Design review of the part built by this model. Coordinates are the model's own, in mm. Face numbers are marked on the shaded views. A direction names the side the tool comes from. Coordinates: 2 decimals unless noted, no trailing zeros. Write each loop counter-clockwise with the first axis right and the second up, starting at its lowest first coordinate (ties: lowest second). Pieces come first, ordered by that corner, then holes. Notation, with made-up numbers: (85.25, 22.5) - (96.25, 22.5) arc R18 cw to (96.25, 39.5) - close; hole circle Ø8 at (-30.75, -12). An arc over 180 degrees is marked (long way). One line per item, written item: value.
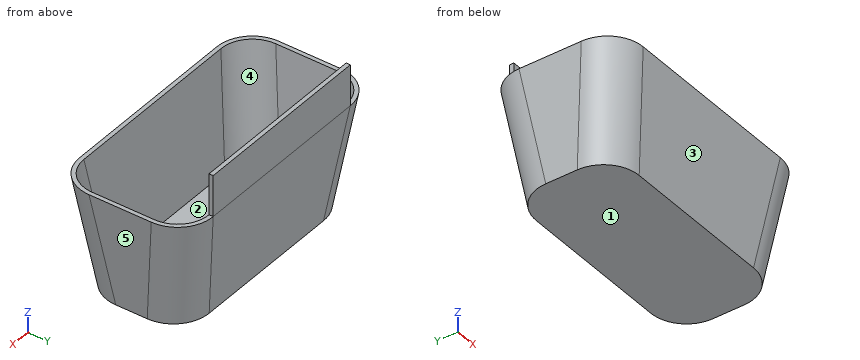
from build123d import *

# Parameters (mm, degrees)
F0_W      = 125
F0_H      = 110
F1_DEPTH  = 65
F3_DEPTH  = 65.001
F5_DEPTH  = 125.001
F8_R      = 35
F9_T      = -4
F10_W     = 180.6418882369
F10_H     = 4.0370187838
F11_DEPTH = 40


with BuildPart() as f1:
    # F0 (on Front) → F1 (new body)
    with BuildSketch(Plane.XZ):
        with Locations((-62.5, 0)):
            Rectangle(F0_W, F0_H)
    extrude(amount=F1_DEPTH)

    # F2 (on face) → F3 (cut, through all)
    with BuildSketch(Plane.XZ.offset(65)):
        Polygon((-110, -55), (-125, 55), (-154.2346477509, 55), (-148.0445983784, -67.179696599), (-108.0001720049, -65.150906356), align=None)
    extrude(amount=-F3_DEPTH, mode=Mode.SUBTRACT)

    # F4 (on face) → F5 (cut, through all)
    with BuildSketch(Plane.YZ):
        Polygon((-50, -55), (-65, 55), (-101.2629643083, 55), (-94.3923816085, -57.4389097095), (-50, -57.4389097095), align=None)
    extrude(amount=-F5_DEPTH, mode=Mode.SUBTRACT)

    # F6: F1 across face


with BuildPart() as f1_1:
    add(f1.part)
    add(f1.part.mirror(Plane(origin=(0, -28.9130434783, 2.3913043478), x_dir=(0, 1, 0), z_dir=(1, 0, 0))))

    # F7: F1 across face


with BuildPart() as f1_2:
    add(f1_1.part)
    add(f1_1.part.mirror(Plane(origin=(0, 0, 1.170212766), x_dir=(-1, 0, 0), z_dir=(0, 1, 0))))

    # F8
    f8_edges = [f1_2.edges().sort_by_distance(p)[0] for p in [
        (-117.5, -57.5, 0),
        (-117.5, 57.5, 0),
        (117.5, -57.5, 0),
        (117.5, 57.5, 0),
    ]]
    fillet(f8_edges, radius=F8_R)

    # F9
    f9_openings = [f1_2.faces().sort_by_distance(p)[0] for p in [
        (0, 0, 55),
    ]]
    offset(amount=F9_T, openings=f9_openings)

    # F10 (on face) → F11 (join)
    with BuildSketch(Plane.XY.offset(55)):
        with Locations((0, 62.9814906081)):
            Rectangle(F10_W, F10_H)
    extrude(amount=F11_DEPTH)


solid = f1_2.part
1. Mouldability with a two-part tool opening along Y and no side actions: class the marked faces 3, 4 and 5 as released by +Y, released by -Y, zero draft, split by the parting line, or undercut.
Answer block:
face 3: released by -Y
face 4: undercut
face 5: zero draft
2. Consider section B-B, the plane z = 61. Write out the cut boundary in (x, y), then the cut area to 3 significant figures.
Answer block:
outline: (-90.32, 60.96) - (90.32, 60.96) - (90.32, 65) - (-90.32, 65) - close
area: 729 mm^2
3. Insertion check: pin 1 Ø2 at (y, z) = (-6, 42) entering from +X; pin 2 Ø3 at (y, z) = (63, 72.5) entering from -X; pin 3 Ø4.5 at (y, z) = (62.5, 71) entering from +X. Each pin has a flat end and moves straight along its axis. Give the tip position at first contact, or say it passes through.
Answer block:
pin 1: stops at x = 123.36
pin 2: stops at x = -90.32
pin 3: stops at x = 90.32
4. Consider section A-A, the plane x = 12. Write out the cut boundary in (y, z), then the cut area to 3 significant figures.
Answer block:
outline: (-65, 55) - (-50, -55) - (50, -55) - (65, 55) - (65, 95) - (60.96, 95) - (60.96, 55) - (46.51, -51) - (-46.51, -51) - (-60.96, 55) - close
area: 1,420 mm^2
5. For the marked faces 1 and 2, list the 3-axis set-ups (+Z, -Z, +X, -X, +Y, -Y) from which the entire face can be reached by the end or side of a thin tool; tool diameter is ignored.
Answer block:
face 1: -Z, +X, -X, +Y, -Y
face 2: +Z
6. Wall thickness on line 1 along Z through (x, y) = (77, -43); line 2 along Y through (x, z) = (-73, -26); line 3 along X through (y, z) = (35.5, 27.5): over which ranges is each line inside the solid? List them lowest first.
Answer block:
line 1: z = -55 to -51
line 2: y = -53.95 to -49.92, 49.92 to 53.95
line 3: x = -120.1 to -115.88, 115.88 to 120.1
